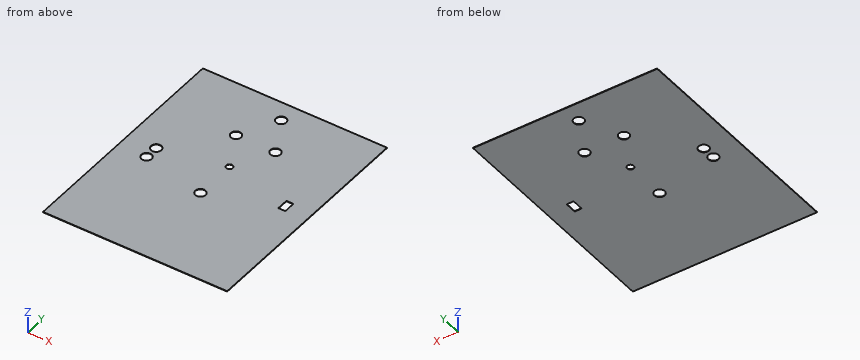
from build123d import *

# Parameters (mm, degrees)
F0_W     = 395
F0_H     = 495
F0_R     = 11
F0_R_2   = 7
F0_W_2   = 15
F0_H_2   = 25
F1_DEPTH = 1


with BuildPart() as f1:
    # F0 (on Top) → F1 (new body)
    with BuildSketch(Plane.XY):
        Rectangle(F0_W, F0_H)
        with Locations((-136.41675, -15)):
            Circle(F0_R, mode=Mode.SUBTRACT)
        with Locations((0, -45)):
            Circle(F0_R, mode=Mode.SUBTRACT)
        with Locations((-136.41675, 15)):
            Circle(F0_R, mode=Mode.SUBTRACT)
        with Locations((-41.486505, 125)):
            Circle(F0_R, mode=Mode.SUBTRACT)
        with Locations((0, 45)):
            Circle(F0_R_2, mode=Mode.SUBTRACT)
        with Locations((145, 10)):
            Rectangle(F0_W_2, F0_H_2, mode=Mode.SUBTRACT)
        with Locations((43.16403, 125)):
            Circle(F0_R, mode=Mode.SUBTRACT)
        with Locations((0, 205)):
            Circle(F0_R, mode=Mode.SUBTRACT)
    extrude(amount=F1_DEPTH)


solid = f1.part
Here's how the part is built. I have some questions about the finished solid (model axes, mm). Give positions to 0.01 mm unless a question says otherwise; leave off trailing zeros. Order: outer loops, then holes, each group sorted by start corner. A loop starts at its lowest first (then second) coordinate and runs counter-clockwise, first axis right, second up. Notation, with made-up numbers: (76, 44.5) -> (81, 44.5) arc R19 cw to (81, 51.5) -> close; hole circle Ø7 at (0, 70). An arc over 180 degrees is marked (long way). Use a Markdown table: item, result. Add a question column.
Item 1: Imagine slicing it at A-A on x = 0. Please give me the cut outline in (y, z), plus the area to 3 significant figures.
Item 2: Imagine slicing it at B-B on y = 125. Please give me the cut outline in (x, z).
Item 3: Imagine slicing it at D-D on y = 205. Please give me the cut outline in (x, z), plus the area to 3 significant figures.
Item 4: Imagine slicing it at C-C on y = 45. Please give me the cut outline in (x, z).
Item 5: I need wall thicknesses on line 1 (Y direction, x = 0, z = 0.45); line 2 (Y direction, x = -6, z = 0.85); line 3 (Y direction, x = 42, z = 0.25). Which ranges of each line are inside material? Lowest first, please.
Data:
| question | item | result |
|---|---|---|
| 1 | outline | (-247.5, 0) -> (-56, 0) -> (-56, 1) -> (-247.5, 1) -> close; (-34, 0) -> (38, 0) -> (38, 1) -> (-34, 1) -> close; (52, 0) -> (194, 0) -> (194, 1) -> (52, 1) -> close; (216, 0) -> (247.5, 0) -> (247.5, 1) -> (216, 1) -> close |
| 1 | area | 437 mm² |
| 2 | outline | (-197.5, 0) -> (-52.49, 0) -> (-52.49, 1) -> (-197.5, 1) -> close; (-30.49, 0) -> (32.16, 0) -> (32.16, 1) -> (-30.49, 1) -> close; (54.16, 0) -> (197.5, 0) -> (197.5, 1) -> (54.16, 1) -> close |
| 3 | outline | (-197.5, 0) -> (-11, 0) -> (-11, 1) -> (-197.5, 1) -> close; (11, 0) -> (197.5, 0) -> (197.5, 1) -> (11, 1) -> close |
| 3 | area | 373 mm² |
| 4 | outline | (-197.5, 0) -> (-7, 0) -> (-7, 1) -> (-197.5, 1) -> close; (7, 0) -> (197.5, 0) -> (197.5, 1) -> (7, 1) -> close |
| 5 | line 1 | y = -247.5 to -56, -34 to 38, 52 to 194, 216 to 247.5 |
| 5 | line 2 | y = -247.5 to -54.22, -35.78 to 41.39, 48.61 to 195.78, 214.22 to 247.5 |
| 5 | line 3 | y = -247.5 to 114.06, 135.94 to 247.5 |
